Geometry check sheet. Reference: drawing and pictorial views, mm from the part's lowest x, y, z. A direction names the side the tool comes from. Round coordinates to 2 decimals unless told otherwise and drop trailing zeros. Loops run counter-clockwise (first coordinate to the right, second up) from the corner with the lowest first, then second, coordinate; pieces in that order, holes last. Notation, with made-up numbers: (-24.75, 75) - (-7.75, 75) arc R23 cw to (-7.75, 109) - close; hole circle Ø5 at (28, -14.5). An arc over 180 degrees is marked (long way). Return JSON: item names as keys, results as strings.
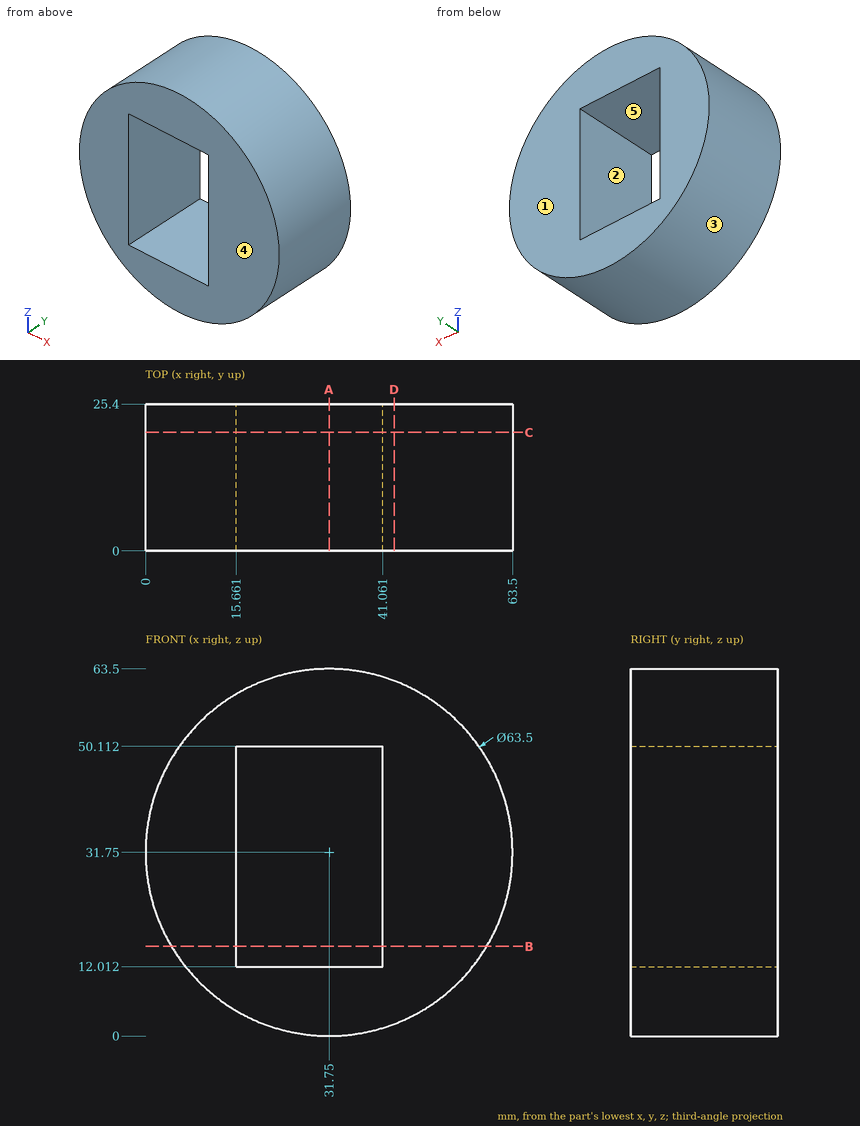
Q1. Sectioned sample at A-A (x = 31.75). Enter the section's corners in (y, z), plus the area to 3 significant figures.
Answer key:
{"outline": "(0, 0) - (25.4, 0) - (25.4, 12.01) - (0, 12.01) - close; (0, 50.11) - (25.4, 50.11) - (25.4, 63.5) - (0, 63.5) - close", "area": "645 mm²"}
Q2. Scan lines: probe 1 along X at (y, z) = (8.75, 31); probe 2 along X at (y, z) = (3.5, 45); probe 3 along Z at (x, y) = (22, 18.5) (1 decimal). Record each from-to range of solid material in increasing order. Write a range as [from, to].
Answer key:
{"probe 1": "x = [0.01, 15.66], [41.06, 63.49]", "probe 2": "x = [2.9, 15.66], [41.06, 60.6]", "probe 3": "z = [1.5, 12], [50.1, 62]"}
Q3. Depth check by flat-ended pin: P1, Ø12.5, axis at x = 24, y = 8.5, coming from the -Z side (1 decimal); P2, Ø10, axis at y = 20, z = 26.5, coming from the -X side; P3, Ø2, axis at x = 15, y = 13.5, coming from the -Z side. Enter the tip coordinate at first touch or a pass-through.
Answer key:
{"P1": "stops at z = 0", "P2": "stops at x = 0", "P3": "stops at z = 4.18"}
Q4. Tool access check on the marked faces 4 and 5. Record the directions out of +Z, -Z, +X, -X, +Y, -Y that give a thin tool (end or side, any length) a straight path to the whole face; none if there is none.
Answer key:
{"face 4": "+Z, -Z, +X, -X, -Y", "face 5": "+Y, -Y"}
Q5. Sectioned sample at C-C (y = 20.5). Enter the section's corners in (x, z).
Answer key:
{"outline": "circle Ø63.5 at (31.75, 31.75); hole (15.66, 12.01) - (41.06, 12.01) - (41.06, 50.11) - (15.66, 50.11) - close"}
Q6. Sectioned sample at D-D (x = 43). Enter the section's corners in (y, z), plus the area to 3 significant figures.
Answer key:
{"outline": "(0, 2.06) - (25.4, 2.06) - (25.4, 61.44) - (0, 61.44) - close", "area": "1,510 mm²"}
Q7. Sectioned sample at B-B (z = 15.5). Enter the section's corners in (x, y).
Answer key:
{"outline": "(4.47, 0) - (15.66, 0) - (15.66, 25.4) - (4.47, 25.4) - close; (41.06, 0) - (59.03, 0) - (59.03, 25.4) - (41.06, 25.4) - close"}
Q8. Draft check along X on the marked faces 1, 2 and 3. Enter one of: released by +X, released by -X, zero draft, split by the parting line, or undercut.
Answer key:
{"face 1": "zero draft", "face 2": "undercut", "face 3": "split by the parting line"}
